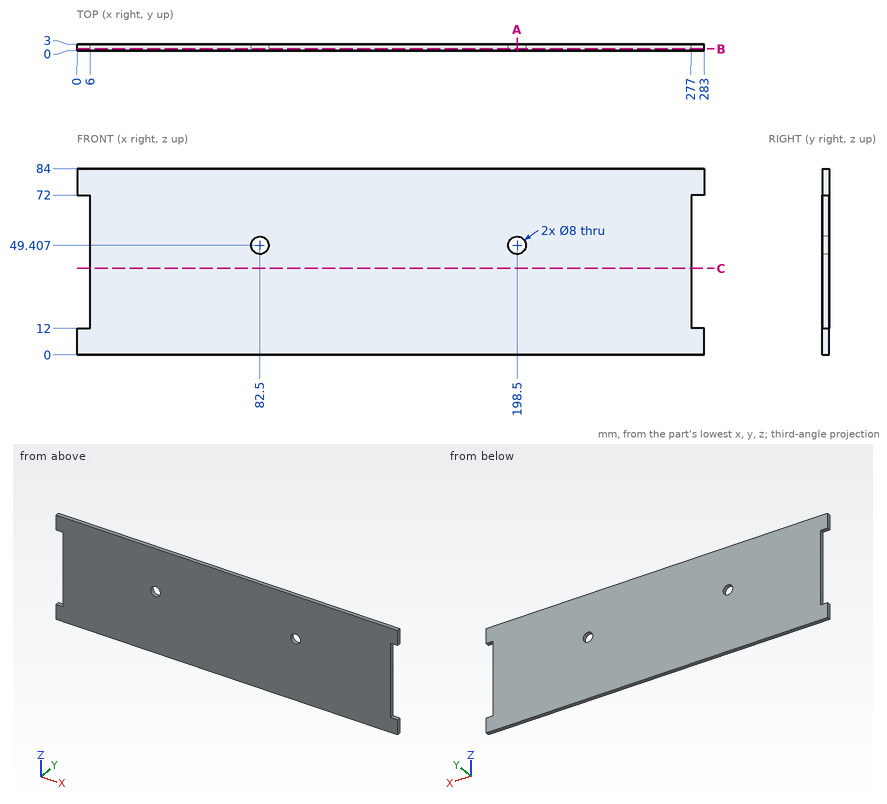
The drawing under review shows one solid part. Ordinate dimensions are in mm from its lowest x, y, z. Coordinates: 2 decimals unless noted, no trailing zeros. Loops run counter-clockwise (first coordinate to the right, second up) from the corner with the lowest first, then second, coordinate; pieces in that order, holes last. Notation, with made-up numbers: M 78,45.5 L 87,45.5 A24 ccw 87,80.5 Z; hole C 80,84 d8. An arc over 180 degrees is marked long. Use one line per item in the form item = value.
(1) Consider section C-C (z = 39). Write out the cut boundary in (x, y), and give its area (3 significant figures).
Return value:
outline = M 6,0 L 277,0 L 277,3 L 6,3 Z
area = 813 mm2
(2) For line 1 along X through (y, z) = (0.65, 49.5); line 2 along X through (y, z) = (1.45, 50.5); line 3 along Z through (x, y) = (82.5, 1.05), list the stretches that pass through material, from the lowest coordinate up. Write a range as from..to.
Return value:
line_1 = 6..78.5, 86.5..194.5, 202.5..277
line_2 = 6..78.65, 86.35..194.65, 202.35..277
line_3 = 0..45.41, 53.41..84
(3) Clearance check with a flat-ended pin moving along its axis: P1, Ø5, axis at x = 82.5, z = 49.407, coming from the +Y side. State where the tip first meets the part, or that it passes through.
Return value:
P1 = through
(4) Consider section A-A (x = 198.5). Write out the cut boundary in (y, z), and give its area (3 significant figures).
Return value:
outline = M 0,0 L 3,0 L 3,45.41 L 0,45.41 Z; M 0,53.41 L 3,53.41 L 3,84 L 0,84 Z
area = 228 mm2
(5) Consider section B-B (y = 0.75). Write out the cut boundary in (x, z).
Return value:
outline = M 0,0 L 283,0 L 283,12 L 277,12 L 277,72 L 283,72 L 283,84 L 0,84 L 0,72 L 6,72 L 6,12 L 0,12 Z; hole C 82.5,49.41 d8; hole C 198.5,49.41 d8
